Can you work these out from the model? Positions are in its coordinate system, mm. Face numbers are marked on the shaded views. A direction names the side the tool comes from. Round coordinates to 2 decimals unless told otherwise and drop trailing zeros. Write each loop counter-clockwise with the first axis right and the second up, starting at its lowest first coordinate (ties: lowest second). Pieces come first, ordered by that corner, then holes. Notation, with made-up numbers: M 9.25,-33 L 33.25,-33 A29 cw 33.25,-2 Z; hole C -10,12 d11. An arc over 180 degrees is marked long. Answer in a Markdown table with one row per item. Add a question column.
(1) Suppose I cut it at B-B, the plane x = 0. Write out the boundary of the cut face in (y, z), then the cut area to 3 significant figures.
(2) Suppose I cut it at A-A, the plane z = 8.25. Count the separate pieces of the cut face and the enclosed holes in it, then the cut area to 3 significant figures.
(3) I'm going to push flat-ended pins straight in: pin 1 (16 mm diameter, centred on x = 40, y = -70, fed in from +Z); pin 2 (5 mm diameter, centred on x = 29, z = 2, fed in from -Y); pin 3 (5 mm diameter, centred on y = 16, z = -1.5, fed in from +X); pin 4 (1 mm diameter, centred on y = -10.5, z = 6.5, fed in from +X). Where does each tip first touch, or does it pass through?
(4) Suppose I cut it at D-D, the plane y = 20. Write out the boundary of the cut face in (x, z), then the cut area to 3 significant figures.
(5) If we mould it in two halves opening along X, with no side actions, what happens to the marked faces 5, 6 and 7? For each: released by +X, released by -X, zero draft, split by the parting line, or undercut.
(6) For the marked faces 1, 2, 3 and 4, which set-ups out of +Z, -Z, +X, -X, +Y, -Y let a thin tool reach every point of the face, with its end or its side?
(7) Suppose I cut it at C-C, the plane x = -20. Write out the boundary of the cut face in (y, z).
(8) If I drill on probe 1 along Y at (x, z) = (0, 6.25); probe 2 along Y at (x, z) = (-40, 5); probe 3 along Y at (x, z) = (3, -8.5), over which ranges is the centre line in solid material (lowest first)?
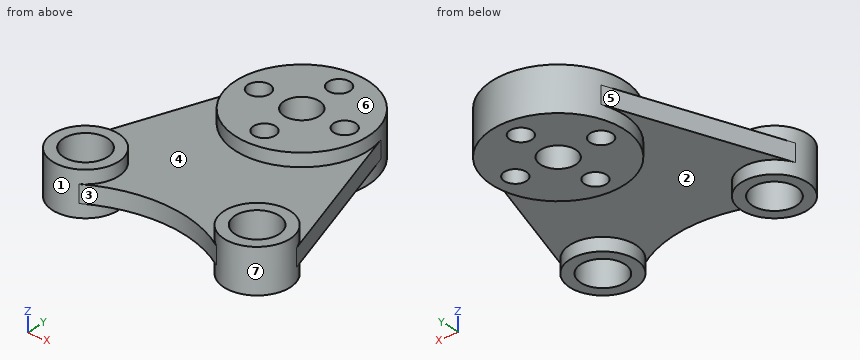
from build123d import *

# Parameters (mm, degrees)
SKETCH1_R             = 30
SKETCH1_R_2           = 8
SKETCH1_R_3           = 5
BOSS_EXTRUDE1_DEPTH   = 10
SKETCH1_R_4           = 15
SKETCH1_R_5           = 10
BOSS_EXTRUDE1_2_DEPTH = 10
BOSS_EXTRUDE1_3_DEPTH = 10
BOSS_EXTRUDE2_DEPTH   = 4


with BuildPart() as part:
    # Sketch1 → Boss-Extrude1 (new, symmetric)
    with BuildSketch(Plane.XY):
        Circle(SKETCH1_R)
        Circle(SKETCH1_R_2, mode=Mode.SUBTRACT)
        with Locations((20, 0)):
            Circle(SKETCH1_R_3, mode=Mode.SUBTRACT)
        with Locations((0, -20)):
            Circle(SKETCH1_R_3, mode=Mode.SUBTRACT)
        with Locations((-20, 0)):
            Circle(SKETCH1_R_3, mode=Mode.SUBTRACT)
        with Locations((0, 20)):
            Circle(SKETCH1_R_3, mode=Mode.SUBTRACT)
    extrude(amount=BOSS_EXTRUDE1_DEPTH, both=True)



with BuildPart() as body_2:
    # Sketch1 → Boss-Extrude1 2 (new, symmetric)
    with BuildSketch(Plane.XY):
        with Locations((40, -70)):
            Circle(SKETCH1_R_4)
        with Locations((40, -70)):
            Circle(SKETCH1_R_5, mode=Mode.SUBTRACT)
    extrude(amount=BOSS_EXTRUDE1_2_DEPTH, both=True)


with BuildPart() as body_3:
    # Sketch1 → Boss-Extrude1 3 (new, symmetric)
    with BuildSketch(Plane.XY):
        with Locations((-40, -70)):
            Circle(SKETCH1_R_4)
        with Locations((-40, -70)):
            Circle(SKETCH1_R_5, mode=Mode.SUBTRACT)
    extrude(amount=BOSS_EXTRUDE1_3_DEPTH, both=True)


with BuildPart() as part_1:
    add(part.part)

    add(body_2.part)  # Boss-Extrude2 merges body 2

    add(body_3.part)  # Boss-Extrude2 merges body 3
    # Sketch1<3> → Boss-Extrude2 (add, symmetric)
    with BuildSketch(Plane.XY):
        with BuildLine():
            Line((54.180868072, -65.11093253), (28.361736144, 9.778134939))
            ThreePointArc((28.361736144, 9.778134939), (29.587599466, 4.957212709), (30, 0))
            ThreePointArc((30, 0), (-4.957212709, -29.587599466), (-28.361736144, 9.778134939))
            Line((-28.361736144, 9.778134939), (-54.180868072, -65.11093253))
            ThreePointArc((-54.180868072, -65.11093253), (-37.521393646, -55.206200267), (-25, -70))
            ThreePointArc((-25, -70), (-26.866074463, -77.245688373), (-32, -82.68857754))
            ThreePointArc((-32, -82.68857754), (0, -73.442887702), (32, -82.68857754))
            ThreePointArc((32, -82.68857754), (30.683660399, -58.24390301), (54.180868072, -65.11093253))
        make_face()
    extrude(amount=BOSS_EXTRUDE2_DEPTH, both=True)


solid = part_1.part
Calculated:
| question | item | result |
|---|---|---|
| 1 | outline | M -73.44,-4 L -30,-4 L -30,-10 L -25,-10 L -25,10 L -30,10 L -30,4 L -73.44,4 Z; M -15,-10 L -8,-10 L -8,10 L -15,10 Z; M 8,-10 L 15,-10 L 15,10 L 8,10 Z; M 25,-10 L 30,-10 L 30,10 L 25,10 Z |
| 1 | area | 828 mm² |
| 2 | separate pieces | 3 |
| 2 | enclosed holes | 7 |
| 2 | area | 3,100 mm² |
| 3 | pin 1 | through |
| 3 | pin 2 | y = -82.38 |
| 3 | pin 3 | x = 26.79 |
| 3 | pin 4 | x = 28.28 |
| 4 | outline | M -22.36,-10 L -5,-10 L -5,10 L -22.36,10 Z; M 5,-10 L 22.36,-10 L 22.36,10 L 5,10 Z |
| 4 | area | 694 mm² |
| 5 | face 5 | released by -X |
| 5 | face 6 | zero draft |
| 5 | face 7 | undercut |
| 6 | face 1 | none |
| 6 | face 2 | -Z |
| 6 | face 3 | +Z, -Z, -Y |
| 6 | face 4 | +Z |
| 7 | outline | M -76.87,-4 L -22.36,-4 L -22.36,-10 L -5,-10 L -5,10 L -22.36,10 L -22.36,4 L -76.87,4 Z; M 5,-10 L 22.36,-10 L 22.36,10 L 5,10 Z |
| 8 | probe 1 | -30 to -25, -15 to -8, 8 to 15, 25 to 30 |
| 8 | probe 2 | -85 to -80, -60 to -55 |
| 8 | probe 3 | -29.85 to -24, -16 to -7.42, 7.42 to 16, 24 to 29.85 |
